```python
from build123d import *

# Parameters (mm, degrees)
BOSS_EXTRUDE1_DEPTH   = 25
BOSS_EXTRUDE1_2_DEPTH = 25
BOSS_EXTRUDE1_3_DEPTH = 25
BOSS_EXTRUDE1_4_DEPTH = 25
BOSS_EXTRUDE1_5_DEPTH = 25
BOSS_EXTRUDE1_6_DEPTH = 25
BOSS_EXTRUDE2_DEPTH   = 5
SKETCH3_R             = 1.55
SKETCH3_W             = 5.4
SKETCH3_H             = 2
SKETCH3_W_2           = 2
SKETCH3_H_2           = 5.4
CUT_EXTRUDE1_DEPTH    = 5
SKETCH4_R             = 3.1
CUT_EXTRUDE2_DEPTH    = 3


with BuildPart() as part:
    # Sketch1 → Boss-Extrude1 (new body)
    with BuildSketch(Plane(origin=(0, 0, 0), x_dir=(1, 0, 0), z_dir=(0, 1, 0))):
        Polygon((-26.02081528, -11.763455967), (-19.142135624, -18.642135624), (-16.656854249, -18.642135624), (-13.656854249, -15.642135624), (-15.778174593, -13.52081528), (-16.944900782, -12.354089091), (-19.066221126, -14.475409435), (-20.02081528, -13.52081528), (-20.975409435, -12.566221126), (-18.854089091, -10.444900782), (-20.02081528, -9.278174593), (-22.142135624, -7.156854249), (-26.384776311, -11.399494937), align=None)
    extrude(amount=BOSS_EXTRUDE1_DEPTH)



with BuildPart() as body_2:
    # Sketch1 → Boss-Extrude1 2 (new body)
    with BuildSketch(Plane(origin=(0, 0, 0), x_dir=(1, 0, 0), z_dir=(0, 1, 0))):
        Polygon((-3.5, 3), (-3.5, 5.996116817), (-8.989164557, 5.996116817), (-14.363961031, 0.621320344), (-5.878679656, -7.863961031), (-4.018601808, -6.003883183), (-3.5, -6.003883183), (-3.5, -3), (-3.5, -1.35), (-6.5, -1.35), (-6.5, 1.35), (-3.5, 1.35), align=None)
    extrude(amount=BOSS_EXTRUDE1_2_DEPTH)


with BuildPart() as body_3:
    # Sketch1 → Boss-Extrude1 3 (new body)
    with BuildSketch(Plane(origin=(0, 0, 0), x_dir=(1, 0, 0), z_dir=(0, 1, 0))):
        Polygon((-10, -32.642135624), (-11.35, -32.642135624), (-11.35, -29.642135624), (-13.414613988, -29.642135624), (-16.414613988, -29.642135624), (-16.414613988, -35.642135624), (-3.660835443, -35.642135624), (-3.660835443, -29.642135624), (-6.660835443, -29.642135624), (-8.65, -29.642135624), (-8.65, -32.642135624), align=None)
    extrude(amount=BOSS_EXTRUDE1_3_DEPTH)


with BuildPart() as body_4:
    # Sketch1 → Boss-Extrude1 4 (new body)
    with BuildSketch(Plane(origin=(0, 0, 0), x_dir=(1, 0, 0), z_dir=(0, 1, 0))):
        Polygon((7.5, 5.996116817), (7.5, -6.242640687), (14.363961031, 0.621320344), (8.989164557, 5.996116817), align=None)
    extrude(amount=BOSS_EXTRUDE1_4_DEPTH)


with BuildPart() as body_5:
    # Sketch1 → Boss-Extrude1 5 (new body)
    with BuildSketch(Plane(origin=(0, 0, 0), x_dir=(1, 0, 0), z_dir=(0, 1, 0))):
        Polygon((16.944900782, -12.354089091), (19.066221126, -14.475409435), (20.02081528, -13.52081528), (20.975409435, -12.566221126), (18.854089091, -10.444900782), (20.02081528, -9.278174593), (22.142135624, -7.156854249), (26.384776311, -11.399494937), (26.02081528, -11.763455967), (19.142135624, -18.642135624), (16.656854249, -18.642135624), (13.656854249, -15.642135624), (15.778174593, -13.52081528), align=None)
    extrude(amount=BOSS_EXTRUDE1_5_DEPTH)


with BuildPart() as body_6:
    # Sketch1 → Boss-Extrude1 6 (new body)
    with BuildSketch(Plane(origin=(0, 0, 0), x_dir=(1, 0, 0), z_dir=(0, 1, 0))):
        Polygon((8.65, -29.642135624), (8.65, -32.642135624), (10, -32.642135624), (11.35, -32.642135624), (11.35, -29.642135624), (13.414613988, -29.642135624), (16.414613988, -29.642135624), (16.414613988, -35.642135624), (3.660835443, -35.642135624), (3.660835443, -29.642135624), (6.660835443, -29.642135624), align=None)
    extrude(amount=BOSS_EXTRUDE1_6_DEPTH)


with BuildPart() as part_1:
    add(part.part)

    add(body_2.part)  # Boss-Extrude2 merges body 2

    add(body_3.part)  # Boss-Extrude2 merges body 3

    add(body_4.part)  # Boss-Extrude2 merges body 4

    add(body_5.part)  # Boss-Extrude2 merges body 5

    add(body_6.part)  # Boss-Extrude2 merges body 6
    # Sketch2 → Boss-Extrude2 (add)
    with BuildSketch(Plane(origin=(0, 0, 0), x_dir=(-1, 0, 0), z_dir=(0, -1, 0))):
        Polygon((-26.384776311, -11.399494937), (-8.989164557, 5.996116817), (8.989164557, 5.996116817), (26.384776311, -11.399494937), (26.384776311, -35.642135624), (-16.414613988, -35.642135624), (-26.384776311, -35.642135624), align=None)
    extrude(amount=BOSS_EXTRUDE2_DEPTH)

    # Sketch3 → Cut-Extrude1 (cut)
    with BuildSketch(Plane(origin=(0, 0, 0), x_dir=(1, 0, 0), z_dir=(0, 1, 0))):
        with Locations(Location((-21.384776311, -25.642135624, 0), (0, 0, 270))):
            Circle(SKETCH3_R)
        with Locations(Location((0, -23.642135624, 0), (0, 0, 270))):
            Circle(SKETCH3_R)
        with Locations(Location((21.384776311, -25.642135624, 0), (0, 0, 90))):
            Circle(SKETCH3_R)
        with Locations((0.1, 0)):
            Rectangle(SKETCH3_W, SKETCH3_H)
        Polygon((-17.970205615, -10.055992052), (-16.555992052, -11.470205615), (-12.737615434, -7.651828996), (-14.151828996, -6.237615434), align=None)
        with Locations((10, -26.042135624)):
            Rectangle(SKETCH3_W_2, SKETCH3_H_2)
        with Locations((-10, -26.042135624)):
            Rectangle(SKETCH3_W_2, SKETCH3_H_2)
        Polygon((12.737615434, -7.651828996), (14.151828996, -6.237615434), (17.970205615, -10.055992052), (16.555992052, -11.470205615), align=None)
    extrude(amount=-CUT_EXTRUDE1_DEPTH, mode=Mode.SUBTRACT)

    # Sketch4 → Cut-Extrude2 (cut)
    with BuildSketch(Plane(origin=(0, 0, 0), x_dir=(1, 0, 0), z_dir=(0, 1, 0))):
        with Locations(Location((-21.384776311, -25.642135624, 0), (0, 0, 270))):
            Circle(SKETCH4_R)
        with Locations(Location((0, -23.642135624, 0), (0, 0, 270))):
            Circle(SKETCH4_R)
        with Locations(Location((21.384776311, -25.642135624, 0), (0, 0, 270))):
            Circle(SKETCH4_R)
    extrude(amount=-CUT_EXTRUDE2_DEPTH, mode=Mode.SUBTRACT)


solid = part_1.part
```
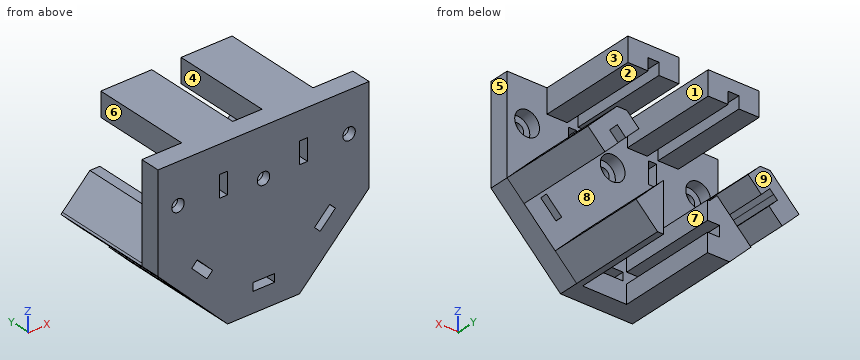
Geometry check sheet. Reference: the model listing, model coordinates, mm. Face numbers are marked on the shaded views. A direction names the side the tool comes from. Round coordinates to 2 decimals unless told otherwise and drop trailing zeros. Order: outer loops, then holes, each group sorted by start corner. A loop starts at its lowest first (then second) coordinate and runs counter-clockwise, first axis right, second up. Notation, with made-up numbers: (20, -20.5) - (58, -20.5) arc R32 cw to (58, 9.5) - close; hole circle Ø10 at (8.5, 36). An arc over 180 degrees is marked (long way). Use a Markdown table: item, result. Add a question column.
1) Mould release check, pull along X, two halves, no side actions. Record for the marked faces 6, 7, 8 and 9: released by +X, released by -X, zero draft, split by the parting line, or undercut.
2) Set-up check for the marked faces 1, 2, 3, 4 and 5: record each of +Z, -Z, +X, -X, +Y, -Y from which the full face is reachable in a straight line by a thin tool's end or side.
3) Section check D-D (z = -2). Record the cut outline in (x, y).
4) Thickness scan on line 1 along Z through (x, y) = (-0.5, -0.25); line 2 along Z through (x, y) = (-7.5, 6.25); line 3 along X through (y, z) = (-1.25, 25). Record the ranges inside material, lowest first.
5) Section check B-B (z = 33.5). Record the cut outline in (x, y), then the cut area to 3 significant figures.
6) Section check C-C (y = 4.5). Count the separate pieces of the cut face and the enclosed holes in it, then the cut area to 3 significant figures.
7) Gauge pin test, flat ends, axial feed: P1, Ø2.5, axis at x = 15, y = 13, coming from the -Z side; P2, Ø1, axis at y = -3.5, z = 0, coming from the +X side; P3, Ø4, axis at y = 20, z = 20.5, coming from the +X side. Record the tip position at first contact, or that the pin passes through.
8) Section check A-A (x = 0). Record the cut outline in (y, z), then the cut area to 3 significant figures.
Established:
| question | item | result |
|---|---|---|
| 1 | face 6 | released by -X |
| 1 | face 7 | undercut |
| 1 | face 8 | undercut |
| 1 | face 9 | zero draft |
| 2 | face 1 | +Z, +Y |
| 2 | face 2 | +X, -X, +Y |
| 2 | face 3 | +Z, +X, +Y |
| 2 | face 4 | +Z, -Z, +Y |
| 2 | face 5 | +Z, -Z, +X, +Y, -Y |
| 3 | outline | (-12.99, -5) - (12.99, -5) - (12.99, 25) - (7.5, 25) - (7.5, 0) - (-3.5, 0) - (-3.5, 25) - (-12.99, 25) - close |
| 4 | line 1 | -6 to -1, 1 to 20.58, 26.7 to 35.64 |
| 4 | line 2 | -6 to 6.24, 29.64 to 35.64 |
| 4 | line 3 | -26.38 to -24.42, -18.35 to -11, -9 to -2.79, 2.79 to 9, 11 to 18.35, 24.42 to 26.38 |
| 5 | outline | (-26.38, -5) - (26.38, -5) - (26.38, 0) - (16.41, 0) - (16.41, 25) - (3.66, 25) - (3.66, 0) - (-3.66, 0) - (-3.66, 25) - (-16.41, 25) - (-16.41, 0) - (-26.38, 0) - close |
| 5 | area | 902 mm2 |
| 6 | separate pieces | 6 |
| 6 | enclosed holes | 0 |
| 6 | area | 397 mm2 |
| 7 | P1 | z = -1.24 |
| 7 | P2 | x = 15.49 |
| 7 | P3 | x = 19.28 |
| 8 | outline | (-5, -6) - (0, -6) - (0, -1) - (-5, -1) - close; (-5, 1) - (0, 1) - (0, 20.54) - (-3, 20.54) - (-3, 22.09) - (-5, 22.09) - close; (-5, 25.19) - (-3, 25.19) - (-3, 26.74) - (0, 26.74) - (0, 35.64) - (-5, 35.64) - close |
| 8 | area | 173 mm2 |
